```python
from build123d import *

# Parameters (mm, degrees)
F0_W        = 4
F0_H        = 12
F1_DEPTH    = 12.2
F2_W        = 2.5
F2_H        = 8.2
F3_DEPTH    = 14.5
F4_W        = 2.5
F4_H        = 8.2
F5_DEPTH    = 13.2
F6_SIZE     = 10
F7_R        = 2
F8_SIZE     = 4
F9_T1_DEPTH = 2
F9_T3_DEPTH = 2
F9_T5_DEPTH = 7.0048288267
F9_T7_DEPTH = 17.2048288267
F9_T9_DEPTH = 7.0048288267


# Not quite as in the source:
# - a fillet or chamfer that OpenCascade refuses, or shapes differently, is made with other operations: its cross-section is extruded or revolved along the edge and cut away or added


with BuildPart() as f1:
    # F0 (on Top) → F1 (new body)
    with BuildSketch(Plane.XY):
        Polygon((-29.984754981, 31.7928069385), (-45.984754981, 31.7928069385), (-45.984754981, 27.7928069385), (-33.984754981, 27.7928069385), (-29.984754981, 27.7928069385), align=None)
        with Locations((-31.984754981, 21.7928069385)):
            Rectangle(F0_W, F0_H)
    extrude(amount=F1_DEPTH)

    # F2 (on face) → F3 (cut)
    with BuildSketch(Plane(origin=(-45.984754981, 0, 0), x_dir=(0, -1, 0), z_dir=(-1, 0, 0))):
        with Locations((-29.0428069385, 6.1)):
            Rectangle(F2_W, F2_H)
    extrude(amount=-F3_DEPTH, mode=Mode.SUBTRACT)

    # F4 (on face) → F5 (cut)
    with BuildSketch(Plane.XZ.offset(-15.7928069385)):
        with Locations((-32.734754981, 6.1)):
            Rectangle(F4_W, F4_H)
    extrude(amount=-F5_DEPTH, mode=Mode.SUBTRACT)

    # F6
    f6_edges = [f1.edges().sort_by_distance(p)[0] for p in [
        (-33.984755, 27.792807, 1),
        (-33.984755, 27.792807, 11.2),
    ]]
    chamfer(f6_edges, length=F6_SIZE)

    # F7
    f7_edges = [f1.edges().sort_by_distance(p)[0] for p in [
        (-31.484755, 30.292807, 6.1),
    ]]
    fillet(f7_edges, radius=F7_R)

    # F8
    f8_edges = [f1.edges().sort_by_distance(p)[0] for p in [
        (-29.984755, 31.792807, 6.1),
    ]]
    chamfer(f8_edges, length=F8_SIZE)

    # F9: fillet of radius 1 on 14 edges, made by hand

    # F9_s2 → F9_t1 (join)
    with BuildSketch(Plane.XY):
        with BuildLine():
            ThreePointArc((-44.3997969705, 27.7932069385), (-44.0161950979, 27.7169037819), (-43.690993133, 27.4996107759))
            Line((-43.690993133, 27.4996107759), (-43.6201127493, 27.5704911597))
            ThreePointArc((-43.6201127493, 27.5704911597), (-43.7671350946, 27.7169478196), (-43.9138745973, 27.8636873222))
            Line((-43.9138745973, 27.8636873222), (-43.984754981, 27.8930469385))
            ThreePointArc((-43.984754981, 27.8930469385), (-44.1922759758, 27.8930469385), (-44.3997969705, 27.8934469385))
            Line((-44.3997969705, 27.8934469385), (-44.3997969705, 27.7932069385))
        make_face()
        with BuildLine():
            ThreePointArc((-34.2779511435, 18.0865687864), (-34.0606581376, 17.7613668216), (-33.984354981, 17.377764949))
            Line((-33.984354981, 17.377764949), (-33.884114981, 17.377764949))
            ThreePointArc((-33.884114981, 17.377764949), (-33.884514981, 17.5852859437), (-33.884514981, 17.7928069385))
            Line((-33.884514981, 17.7928069385), (-33.9138745973, 17.8636873222))
            ThreePointArc((-33.9138745973, 17.8636873222), (-34.0606140999, 18.0104268249), (-34.2070707598, 18.1574491702))
            Line((-34.2070707598, 18.1574491702), (-34.2779511435, 18.0865687864))
        make_face()
    extrude(amount=F9_T1_DEPTH)

    # F9_s4 → F9_t3 (join)
    with BuildSketch(Plane.XY.offset(10.2)):
        with BuildLine():
            ThreePointArc((-44.3997969705, 27.7932069385), (-44.0161950979, 27.7169037819), (-43.690993133, 27.4996107759))
            Line((-43.690993133, 27.4996107759), (-43.6201127493, 27.5704911597))
            ThreePointArc((-43.6201127493, 27.5704911597), (-43.7671350946, 27.7169478196), (-43.9138745973, 27.8636873222))
            Line((-43.9138745973, 27.8636873222), (-43.984754981, 27.8930469385))
            ThreePointArc((-43.984754981, 27.8930469385), (-44.1922759758, 27.8930469385), (-44.3997969705, 27.8934469385))
            Line((-44.3997969705, 27.8934469385), (-44.3997969705, 27.7932069385))
        make_face()
        with BuildLine():
            ThreePointArc((-33.984354981, 17.377764949), (-34.0606581376, 17.7613668216), (-34.2779511435, 18.0865687864))
            Line((-34.2779511435, 18.0865687864), (-34.2070707598, 18.1574491702))
            ThreePointArc((-34.2070707598, 18.1574491702), (-34.0606140999, 18.0104268249), (-33.9138745973, 17.8636873222))
            Line((-33.9138745973, 17.8636873222), (-33.884514981, 17.7928069385))
            ThreePointArc((-33.884514981, 17.7928069385), (-33.884514981, 17.5852859437), (-33.884114981, 17.377764949))
            Line((-33.884114981, 17.377764949), (-33.984354981, 17.377764949))
        make_face()
    extrude(amount=F9_T3_DEPTH)

    # F9_s6 → F9_t5 (cut)
    with BuildSketch(Plane.XY.offset(7.6975855866)):
        with BuildLine():
            ThreePointArc((-45.985154981, 28.7937726239), (-45.6918617622, 28.0857001573), (-44.9837892956, 27.7924069385))
            Line((-44.9837892956, 27.7924069385), (-44.9837892956, 27.6922703699))
            ThreePointArc((-44.9837892956, 27.6922703699), (-45.4842721383, 27.6926703699), (-45.984754981, 27.6926703699))
            Line((-45.984754981, 27.6926703699), (-46.0848915495, 27.7928069385))
            ThreePointArc((-46.0848915495, 27.7928069385), (-46.0848915495, 28.2932897812), (-46.0852915495, 28.7937726239))
            Line((-46.0852915495, 28.7937726239), (-45.985154981, 28.7937726239))
        make_face()
        with BuildLine():
            ThreePointArc((-32.9837892956, 15.7924069385), (-33.6918617622, 16.0857001573), (-33.985154981, 16.7937726239))
            Line((-33.985154981, 16.7937726239), (-34.0852915495, 16.7937726239))
            ThreePointArc((-34.0852915495, 16.7937726239), (-34.0848915495, 16.2932897812), (-34.0848915495, 15.7928069385))
            Line((-34.0848915495, 15.7928069385), (-33.984754981, 15.6926703699))
            ThreePointArc((-33.984754981, 15.6926703699), (-33.4842721383, 15.6926703699), (-32.9837892956, 15.6922703699))
            Line((-32.9837892956, 15.6922703699), (-32.9837892956, 15.7924069385))
        make_face()
    extrude(amount=F9_T5_DEPTH, mode=Mode.SUBTRACT)

    # F9_s8 → F9_t7 (cut)
    with BuildSketch(Plane.XY.offset(-2.5024144134)):
        with BuildLine():
            ThreePointArc((-29.984354981, 16.7937726239), (-30.2776481998, 16.0857001573), (-30.9857206664, 15.7924069385))
            Line((-30.9857206664, 15.7924069385), (-30.9857206664, 15.6922703699))
            ThreePointArc((-30.9857206664, 15.6922703699), (-30.4852378237, 15.6926703699), (-29.984754981, 15.6926703699))
            Line((-29.984754981, 15.6926703699), (-29.8846184125, 15.7928069385))
            ThreePointArc((-29.8846184125, 15.7928069385), (-29.8846184125, 16.2932897812), (-29.8842184125, 16.7937726239))
            Line((-29.8842184125, 16.7937726239), (-29.984354981, 16.7937726239))
        make_face()
        with BuildLine():
            ThreePointArc((-45.985154981, 30.7918412531), (-45.6918617622, 31.4999137197), (-44.9837892956, 31.7932069385))
            Line((-44.9837892956, 31.7932069385), (-44.9837892956, 31.893343507))
            ThreePointArc((-44.9837892956, 31.893343507), (-45.4842721383, 31.892943507), (-45.984754981, 31.892943507))
            Line((-45.984754981, 31.892943507), (-46.0848915495, 31.7928069385))
            ThreePointArc((-46.0848915495, 31.7928069385), (-46.0848915495, 31.2923240958), (-46.0852915495, 30.7918412531))
            Line((-46.0852915495, 30.7918412531), (-45.985154981, 30.7918412531))
        make_face()
    extrude(amount=F9_T7_DEPTH, mode=Mode.SUBTRACT)

    # F9_s10 → F9_t9 (cut)
    with BuildSketch(Plane.XY.offset(-2.5024144134)):
        with BuildLine():
            ThreePointArc((-32.9837892956, 15.7924069385), (-33.6918617622, 16.0857001573), (-33.985154981, 16.7937726239))
            Line((-33.985154981, 16.7937726239), (-34.0852915495, 16.7937726239))
            ThreePointArc((-34.0852915495, 16.7937726239), (-34.0848915495, 16.2932897812), (-34.0848915495, 15.7928069385))
            Line((-34.0848915495, 15.7928069385), (-33.984754981, 15.6926703699))
            ThreePointArc((-33.984754981, 15.6926703699), (-33.4842721383, 15.6926703699), (-32.9837892956, 15.6922703699))
            Line((-32.9837892956, 15.6922703699), (-32.9837892956, 15.7924069385))
        make_face()
        with BuildLine():
            ThreePointArc((-44.9837892956, 27.7924069385), (-45.6918617622, 28.0857001573), (-45.985154981, 28.7937726239))
            Line((-45.985154981, 28.7937726239), (-46.0852915495, 28.7937726239))
            ThreePointArc((-46.0852915495, 28.7937726239), (-46.0848915495, 28.2932897812), (-46.0848915495, 27.7928069385))
            Line((-46.0848915495, 27.7928069385), (-45.984754981, 27.6926703699))
            ThreePointArc((-45.984754981, 27.6926703699), (-45.4842721383, 27.6926703699), (-44.9837892956, 27.6922703699))
            Line((-44.9837892956, 27.6922703699), (-44.9837892956, 27.7924069385))
        make_face()
    extrude(amount=F9_T9_DEPTH, mode=Mode.SUBTRACT)


solid = f1.part
```
Model file for the job. Use its own axes, mm. A direction names the side the tool comes from. Coordinates: 2 decimals unless noted, no trailing zeros. Order: outer loops, then holes, each group sorted by start corner. A loop starts at its lowest first (then second) coordinate and runs counter-clockwise, first axis right, second up. Notation, with made-up numbers: (8.5, 75) -> (42.5, 75) arc R18 cw to (42.5, 85) -> close; hole circle Ø1 at (-13, -14.5). An arc over 180 degrees is marked (long way). Return JSON: item names as keys, results as strings.
Item 1: Slice it at C-C (x = -42.75). Write the cut outline in (y, z).
Model answer:
{"outline": "(26.56, 0) -> (31.79, 0) -> (31.79, 12.2) -> (26.56, 12.2) -> (26.56, 10.2) -> (30.29, 10.2) -> (30.29, 2) -> (26.56, 2) -> close"}
Item 2: Slice it at A-A (z = 4.5). Write the cut outline in (x, y), then the cut area to 3 significant figures.
Model answer:
{"outline": "(-45.98, 30.29) -> (-33.48, 30.29) arc R2 cw to (-31.48, 28.29) -> (-31.48, 15.79) -> (-30.96, 15.79) arc R1 ccw to (-29.98, 16.77) -> (-29.98, 27.79) -> (-33.98, 31.79) -> (-45.01, 31.79) arc R1 ccw to (-45.98, 30.82) -> close", "area": "38.2 mm²"}
Item 3: 3-axis set-ups, long thin cutter, end or side, ignore diameter. For faces 1 (the face through (-37, 25, 2)), 2 (the face through (-30.27, 16.093, 6.015)): which of +Z, -Z, +X, -X, +Y, -Y reach the whole face in a straight line?
Model answer:
{"face 1": "-X, -Y", "face 2": "+Z, -Z, +X, -Y"}
Item 4: Pin check, flat tips, straight feed: P1, Ø0.7, axis at x = -44.5, z = 11.5, coming from the -Y side; P2, Ø2, axis at y = 19, z = 8.5, coming from the -X side; P3, Ø2.5, axis at x = -39.5, z = 4.5, coming from the -Y side. Stop position of each tip, or through.
Model answer:
{"P1": "stops at y = 27.76", "P2": "stops at x = -31.48", "P3": "stops at y = 30.29"}
Item 5: Wall check: line 1 along Z through (x, y) = (-34, 23.5); line 2 along X through (y, z) = (25.25, 4.5); line 3 along Y through (x, z) = (-42.25, 8). Give the ranges that are in metal, low to high. Write a range as from..to.
Model answer:
{"line 1": "z = 0..2, 10.2..12.2", "line 2": "x = -31.48..-29.98", "line 3": "y = 30.29..31.79"}
Item 6: Slice it at B-B (y = 29.5). Write the cut outline in (x, z), then the cut area to 3 significant figures.
Model answer:
{"outline": "(-45.98, 0) -> (-31.69, 0) -> (-31.69, 12.2) -> (-45.98, 12.2) -> (-45.98, 10.2) -> (-31.89, 10.2) -> (-31.89, 2) -> (-45.98, 2) -> close", "area": "58.8 mm²"}
Item 7: Slice it at D-D (z = 10.5). Write the cut outline in (x, y).
Model answer:
{"outline": "(-45.98, 28.77) arc R1 ccw to (-45.01, 27.79) -> (-44.37, 27.79) arc R1 cw to (-43.71, 27.52) -> (-34.26, 18.07) arc R1 cw to (-33.98, 17.41) -> (-33.98, 16.77) arc R1 ccw to (-33.01, 15.79) -> (-30.96, 15.79) arc R1 ccw to (-29.98, 16.77) -> (-29.98, 27.79) -> (-33.98, 31.79) -> (-45.01, 31.79) arc R1 ccw to (-45.98, 30.82) -> close"}
Item 8: Mould opens along Z. For faces 3 (the face through (-31.485, 22, 6)), 4 (the face through (-33.684, 16.078, 0.986)), 5 (the face through (-36, 26, 0)) say: pulls with the +Z half, pulls with the -Z half, needs draft (parallel to the pull), parting line crosses it, or undercut.
Model answer:
{"face 3": "undercut", "face 4": "needs draft", "face 5": "pulls with the -Z half"}
